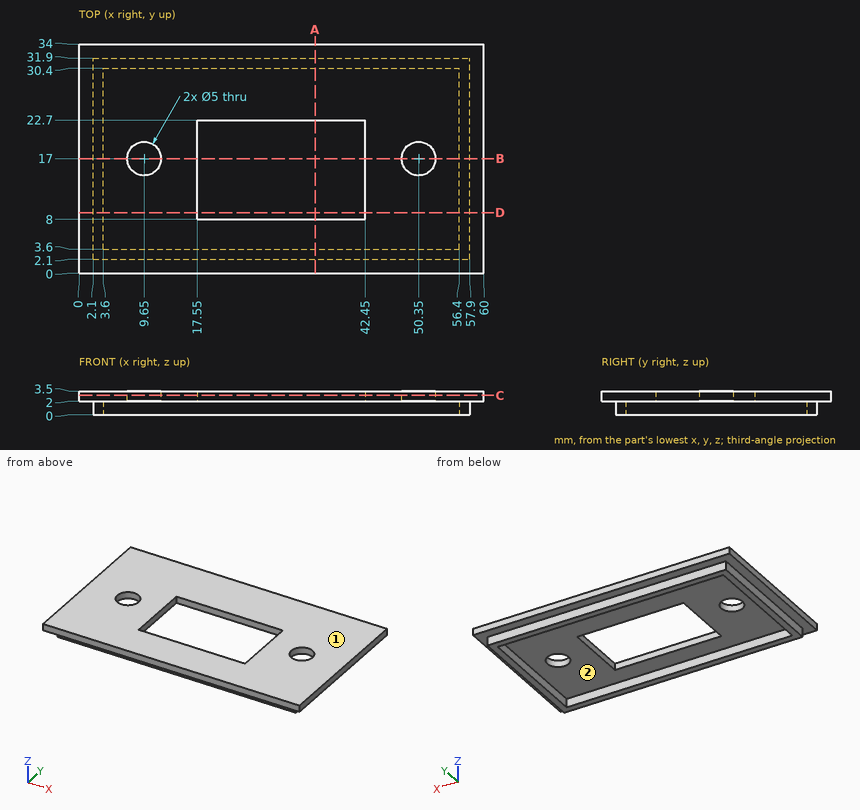
Design review of the part shown in the three views and the two pictorial views. Dimensions are in mm from the part's minimum x, y and z. Give positions to 0.01 mm unless a question says otherwise; leave off trailing zeros. Loops run counter-clockwise (first coordinate to the right, second up) from the corner with the lowest first, then second, coordinate; pieces in that order, holes last. Notation, with made-up numbers: (29.5, 65) -> (60.5, 65) arc R22 cw to (60.5, 93) -> close; hole circle Ø8 at (6, -19.75). An arc over 180 degrees is marked (long way). One line per item, written item: value.
Q1. For pin 1 Ø6 at (x, y) = (9.65, 17) entering from -Z; pin 2 Ø1.6 at (x, z) = (25.5, 1) entering from +Y; pin 3 Ø2 at (x, y) = (20, 11.5) entering from -Z; pin 4 Ø1 at (y, z) = (23, 1) entering from +X, all flat-tipped, find the tip position at first contact; note any pin that passes through.
Numbers:
pin 1: stops at z = 2
pin 2: stops at y = 31.9
pin 3: passes through
pin 4: stops at x = 57.9
Q2. We need section B-B on y = 17. Give the boundary of the cut face in (x, z).
Numbers:
outline: (0, 2) -> (2.1, 2) -> (2.1, 0) -> (3.6, 0) -> (3.6, 2) -> (7.15, 2) -> (7.15, 3.5) -> (0, 3.5) -> close; (12.15, 2) -> (17.55, 2) -> (17.55, 3.5) -> (12.15, 3.5) -> close; (42.45, 2) -> (47.85, 2) -> (47.85, 3.5) -> (42.45, 3.5) -> close; (52.85, 2) -> (56.4, 2) -> (56.4, 0) -> (57.9, 0) -> (57.9, 2) -> (60, 2) -> (60, 3.5) -> (52.85, 3.5) -> close
Q3. We need section D-D on y = 9. Give the boundary of the cut face in (x, z).
Numbers:
outline: (0, 2) -> (2.1, 2) -> (2.1, 0) -> (3.6, 0) -> (3.6, 2) -> (17.55, 2) -> (17.55, 3.5) -> (0, 3.5) -> close; (42.45, 2) -> (56.4, 2) -> (56.4, 0) -> (57.9, 0) -> (57.9, 2) -> (60, 2) -> (60, 3.5) -> (42.45, 3.5) -> close
Q4. We need section A-A on x = 35. Give the boundary of the cut face in (y, z), and give its area (4 significant figures).
Numbers:
outline: (0, 2) -> (2.1, 2) -> (2.1, 0) -> (3.6, 0) -> (3.6, 2) -> (8, 2) -> (8, 3.5) -> (0, 3.5) -> close; (22.7, 2) -> (30.4, 2) -> (30.4, 0) -> (31.9, 0) -> (31.9, 2) -> (34, 2) -> (34, 3.5) -> (22.7, 3.5) -> close
area: 34.95 mm^2
Q5. Draft analysis for pull direction X (two halves, no side actions). For the marked faces 1 and 2, state which applies: pulls with the +X half, pulls with the -X half, needs draft (parallel to the pull), parting line crosses it, or undercut.
Numbers:
face 1: needs draft
face 2: undercut
Q6. We need section C-C on z = 2.9. Give the boundary of the cut face in (x, y), and give its area (3 significant figures).
Numbers:
outline: (0, 0) -> (60, 0) -> (60, 34) -> (0, 34) -> close; hole circle Ø5 at (9.65, 17); hole (17.55, 8) -> (42.45, 8) -> (42.45, 22.7) -> (17.55, 22.7) -> close; hole circle Ø5 at (50.35, 17)
area: 1,630 mm^2
Q7. For L1, parallel to Y at x = 52, z = 1.2; L2, parallel to X at y = 11.5, z = 3.1; L3, parallel to Y at x = 50.35, z = 3.25, list the stretches that pass through material, from the lowest coordinate up.
Numbers:
L1: y = 2.1 to 3.6, 30.4 to 31.9
L2: x = 0 to 17.55, 42.45 to 60
L3: y = 0 to 14.5, 19.5 to 34
